CAD build for the part. Positions are in the model's coordinates, mm. A direction names the side the tool comes from. Give positions to 0.01 mm unless a question says otherwise; leave off trailing zeros. Put each result on its own line as item: value. Start each with the question number.
1) Two-plate mould, pull along Z, no slides. Class faces 1 (the face through (71, 1, 114.3)), 2 (the face through (46, 0, -137.16)), 3 (the face through (181.83, -4, -43)): released by +Z, released by -Z, zero draft, split by the parting line, or undercut.
2) Drill centre lines: line 1 (Z direction, x = 59, y = 1.5); line 2 (Y direction, x = 77.5, z = -38.5) (3 decimals); line 3 (Y direction, x = 116.5, z = -50.8). Where is each one in solid material? Low to high. Write a range as [from, to].
3) Tool access for faces 4 (the face through (38.633, 7.629, -26.573)), 5 (the face through (10.17, 0.45, -126.49)), 6 (the face through (180.401, -7.246, -33.324)): list every direction of +Z, -Z, +X, -X, +Y, -Y with a clear straight run to the whole face (end or side of a thin tool).
4) Pin check, flat tips, straight feed: pin 1 (1.5 mm diameter, centred on x = 115, y = 19.5, fed in from -Z); pin 2 (1 mm diameter, centred on x = 177, z = -18, fed in from -Y); pin 3 (4 mm diameter, centred on x = 68.5, y = -58, fed in from +Z). Stop position of each tip, or through.
```python
from build123d import *

# Parameters (mm, degrees)
F3_R     = 10.16
F4_DEPTH = 35.56


# Not quite as in the source:
# - a feature names something its author has since deleted; it is built from what else it names


with BuildPart() as f1:
    # F0 (on Front) → F1 (revolve)
    with BuildSketch(Plane.XZ):
        with BuildLine():
            Line((207.1336402178, -42.8901373174), (207.1336402178, -32.7301373174))
            add(Edge.make_bspline(
                [(0, 0), (10.4638618624, 8.1276784662), (33.2666475246, 37.2417350062), (163.1452860385, 2.6466282002), (191.1877777142, -17.7927619281), (207.1336402178, -32.7301373174)],
                knots=[0, 0, 0, 0, 0.2590203832, 0.6935859965, 1, 1, 1, 1], degree=3))
            Line((0, 0), (0, -25.4))
            Line((0, -25.4), (76.2, -25.4))
            Line((76.2, -25.4), (76.2, -15.24))
            Line((76.2, -15.24), (152.4, -15.24))
            Line((152.4, -15.24), (181.8301071367, -32.7301373174))
            Line((181.8301071367, -32.7301373174), (181.8301071367, -42.8901373174))
            Line((181.8301071367, -42.8901373174), (207.1336402178, -42.8901373174))
        make_face()
    revolve(axis=Axis((71.7367434391, 0, -50.8), (-1, 0, 0)))

    # F3 (on offset) → F4 (join)
    with BuildSketch(Plane.XY.offset(-101.6)):
        with Locations((20.32, 0)):
            Circle(F3_R)
        with Locations((45.72, 0)):
            Circle(F3_R)
    extrude(amount=-F4_DEPTH)

    # F8: sweep along a path in F5
    with BuildLine(Plane.XZ) as f8_path:
        add(Plane.XZ * Edge.make_bspline(
            [(39.8880077945, 0), (54.9183498543, 38.4224136512), (76.2580250899, 92.973522723), (73.0281734091, 109.4334294306), (72.0732286811, 114.3)],
            knots=[0, 0, 0, 0, 0.7043379008, 1, 1, 1, 1], degree=3))
    # F7 (on offset) → F8 (sweep)
    with BuildSketch(Plane.XY.offset(114.3)):
        with BuildLine():
            add(Edge.make_bspline(
                [(53.0232286811, 0), (53.0232286811, -15.3979316793), (81.5982286811, -7.6989658396), (110.1732286811, 0), (81.5982286811, 7.6989658396), (53.0232286811, 15.3979316793), (53.0232286811, 0)],
                knots=[0, 0, 0, 2.0943951024, 2.0943951024, 4.1887902048, 4.1887902048, 6.2831853072, 6.2831853072, 6.2831853072], degree=2, weights=[1, 0.5, 1, 0.5, 1, 0.5, 1]))
        make_face()
    sweep(path=f8_path.line)


solid = f1.part
```
Solution:
1. face 1: released by +Z
1. face 2: released by -Z
1. face 3: undercut
2. line 1: [-125.16, -76.16], [-25.44, 114.3]
2. line 2: [-71.408, -33.365], [33.365, 71.408]
2. line 3: [-64.05, -35.56], [35.56, 64.05]
3. face 4: -X
3. face 5: -Z
3. face 6: none
4. pin 1: z = -112.55
4. pin 2: y = -25.54
4. pin 3: z = -3
